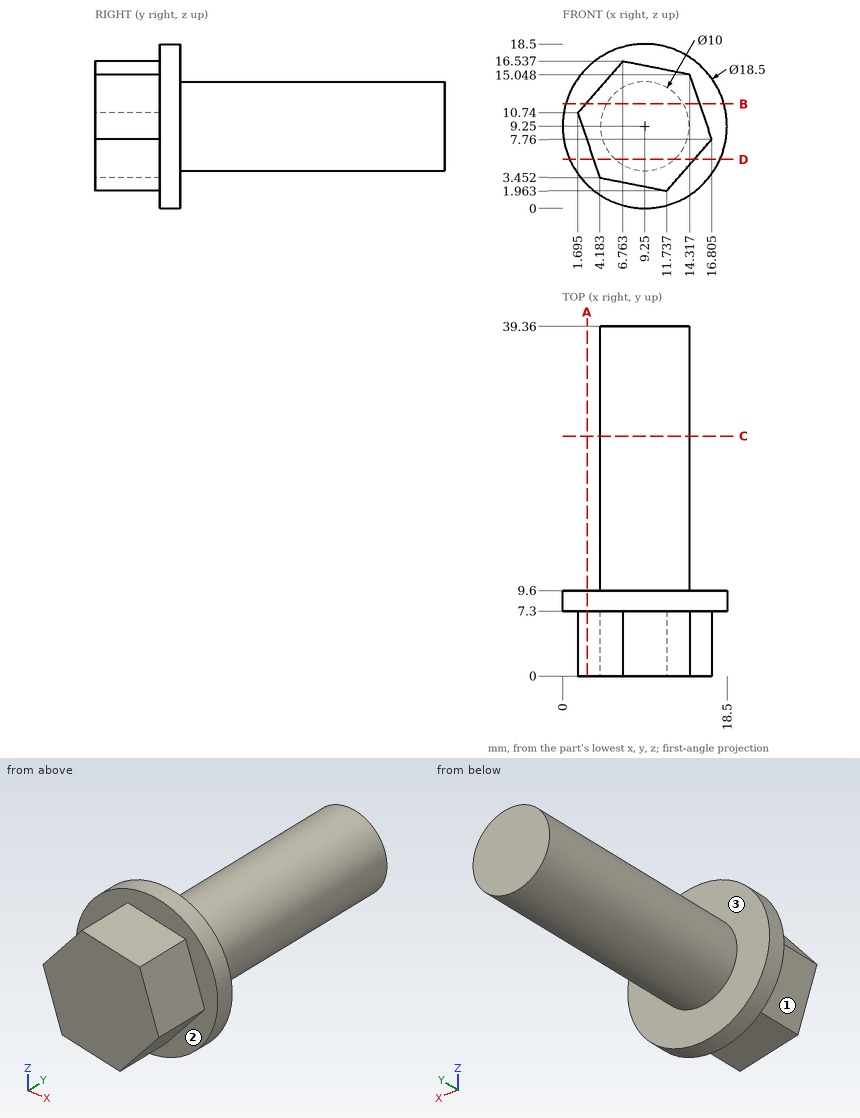
Study the drawing (mm; zero at the part's minimum x, y, z) and answer. A direction names the side the tool comes from. Give positions to 0.01 mm unless a question says otherwise; leave off trailing zeros. Write each loop counter-clockwise with the first axis right and the second up, starting at its lowest first coordinate (ties: lowest second). Pieces come first, ordered by that corner, then holes. Notation, with made-up numbers: (-18, -4.5) -> (-6, -4.5) arc R23 cw to (-6, 8.5) -> close; hole circle Ø2 at (71.5, -8). An arc over 180 degrees is marked (long way). Write item = value, one per line.
Q1. Section A-A on x = 2.75 is taken. Determine the outline of the cut face in (y, z).
Computed values:
outline = (0, 7.65) -> (7.3, 7.65) -> (7.3, 2.67) -> (9.6, 2.67) -> (9.6, 15.83) -> (7.3, 15.83) -> (7.3, 11.95) -> (0, 11.95) -> close
Q2. A tool of negligible diameter and unlimited length cuts with its end or side. For the marked faces 1, 2 and 3, from which of +Z, -Z, +X, -X, +Y, -Y can it reach the whole face along a straight path? Write none if from no direction.
Computed values:
face_1 = -Z, -X, -Y
face_2 = -Y
face_3 = +Y
Q3. Flat-ended cylindrical pins translate along their axes: pin 1 Ø2 at (x, z) = (4.5, 14.5) entering from +Y; pin 2 Ø8 at (y, z) = (9, 5) entering from -X; pin 3 Ø5 at (y, z) = (29, 5.5) entering from -X. Find the tip coordinate at first contact, or state that the pin passes through.
Computed values:
pin_1 = 9.6
pin_2 = 0
pin_3 = 4.41
Q4. Section C-C on y = 27 is taken. Determine the outline of the cut face in (x, z).
Computed values:
outline = circle Ø10 at (9.25, 9.25)
Q5. Section D-D on z = 5.5 is taken. Determine the outline of the cut face in (x, y) (1 decimal).
Computed values:
outline = (0.8, 7.3) -> (3.5, 7.3) -> (3.5, 0) -> (14.8, 0) -> (14.8, 7.3) -> (17.7, 7.3) -> (17.7, 9.6) -> (12.6, 9.6) -> (12.6, 39.4) -> (5.9, 39.4) -> (5.9, 9.6) -> (0.8, 9.6) -> close
Q6. Section B-B on z = 11.75 is taken. Determine the outline of the cut face in (x, y) (1 decimal).
Computed values:
outline = (0.3, 7.3) -> (2.6, 7.3) -> (2.6, 0) -> (15.4, 0) -> (15.4, 7.3) -> (18.2, 7.3) -> (18.2, 9.6) -> (13.6, 9.6) -> (13.6, 39.4) -> (4.9, 39.4) -> (4.9, 9.6) -> (0.3, 9.6) -> close
Q7. Consider line 1 along Y through (x, z) = (15, 3); line 2 along X through (y, z) = (26, 9); line 3 along Y through (x, z) = (15, 9.5). Determine where each line is inside the solid, lowest interval first.
Computed values:
line_1 = 7.3 to 9.6
line_2 = 4.26 to 14.24
line_3 = 0 to 9.6
